For this review, take the finished solid that the model builds, in its own axes (mm). Coordinates: 2 decimals unless noted, no trailing zeros. Loops run counter-clockwise (first coordinate to the right, second up) from the corner with the lowest first, then second, coordinate; pieces in that order, holes last. Notation, with made-up numbers: (21, 58.25) - (25, 58.25) arc R19 ccw to (25, 63.25) - close; hole circle Ø11 at (59.25, 34). An arc over 180 degrees is marked (long way). Use one line per item in the form item = value. Start each with the question number.
1. Add section D-D on y = -90. Give the boundary of the cut face in (x, z), and give its area (3 significant figures).
2. Add section A-A on y = -63.5. Give the boundary of the cut face in (x, z).
3. To check wall thickness, follow probe 1 along Z at (x, y) = (1, -35); probe 2 along Z at (x, y) = (-0.5, -34.5); probe 3 along X at (y, z) = (-93, -73). State the ranges of each line that lie inside material, in increasing order.
4. For pin 1 Ø5 at (x, y) = (1, -5.5) entering from +Z; pin 2 Ø1.7 at (x, z) = (7.5, -75) entering from +Y, all flat-tipped, find the tip position at first contact; note any pin that passes through.
5. Add section B-B on z = -117.5. Give the boundary of the cut face in (x, y).
```python
from build123d import *


with BuildPart() as part:
    # Sweep3: sweep along a path in Sketch3
    with BuildLine(Plane(origin=(0, 0, 0), x_dir=(0, 0, -1), z_dir=(1, 0, 0))) as sweep3_path:
        Line((0, 0), (-7.1374, 0))
        ThreePointArc((-7.1374, 0), (-16.117656121, -3.719743879), (-19.8374, -12.7))
        Line((-19.8374, -12.7), (-19.8374, -82.55))
        ThreePointArc((-19.8374, -82.55), (-16.117656121, -91.530256121), (-7.1374, -95.25))
        Line((-7.1374, -95.25), (145.2626, -95.25))
        ThreePointArc((145.2626, -95.25), (154.242856121, -91.530256121), (157.9626, -82.55))
        Line((157.9626, -82.55), (157.9626, -12.7))
        ThreePointArc((157.9626, -12.7), (154.242856121, -3.719743879), (145.2626, 0))
        Line((145.2626, 0), (138.1252, 0))
    # Sketch2 → Sweep3 (sweep)
    with BuildSketch(Plane.XY):
        Polygon((0, 0), (6.35, 0), (6.35, -7.9375), (7.9375, -7.9375), (7.9375, 1.5875), (-1.5875, 1.5875), (-1.5875, -7.9375), (0, -7.9375), align=None)
    sweep(path=sweep3_path.line)


solid = part.part
```
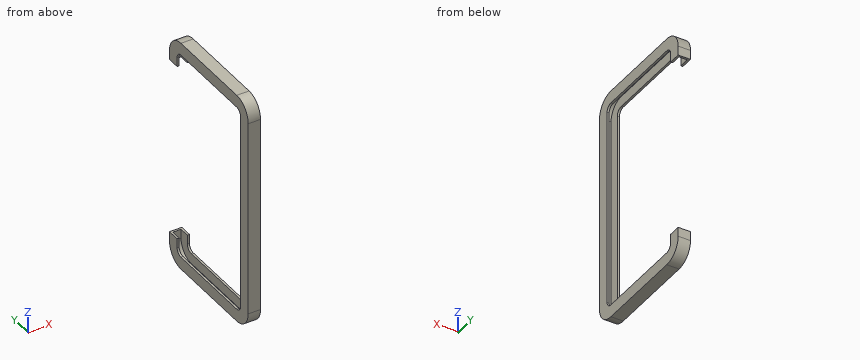
Conclusion:
q1.outline = (-1.59, -157.45) - (7.94, -157.45) - (7.94, 19.33) - (-1.59, 19.33) - close; hole (0, -155.55) - (6.35, -155.55) - (6.35, 17.42) - (0, 17.42) - close
q1.area = 585 mm^2
q2.outline = (-1.59, -159.55) - (7.94, -159.55) - (7.94, -150.03) - (6.35, -150.03) - (6.35, -157.96) - (0, -157.96) - (0, -150.03) - (-1.59, -150.03) - close; (-1.59, 11.9) - (0, 11.9) - (0, 19.84) - (6.35, 19.84) - (6.35, 11.9) - (7.94, 11.9) - (7.94, 21.42) - (-1.59, 21.42) - close
q3.probe_1 = -159.55 to -157.96, 19.84 to 21.42
q3.probe_2 = -159.55 to -150.03, 11.9 to 21.42
q3.probe_3 = -1.59 to 0, 6.35 to 7.94
q4.pin_1 = 20.63
q4.pin_2 = -87.31
q5.outline = (-1.59, -96.84) - (7.94, -96.84) - (7.94, -87.31) - (6.35, -87.31) - (6.35, -95.25) - (0, -95.25) - (0, -87.31) - (-1.59, -87.31) - close
